Read the model definition and answer for the solid it produces. Units are mm, in the model's axes. Face numbers are marked on the shaded views. Coordinates: 2 decimals unless noted, no trailing zeros. Order: outer loops, then holes, each group sorted by start corner. A loop starts at its lowest first (then second) coordinate and runs counter-clockwise, first axis right, second up. Notation, with made-up numbers: M 87,-27.75 L 116,-27.75 A16 ccw 116,-12.75 Z; hole C -15,-17 d5. An arc over 180 degrees is marked long. Put each result on its own line as item: value.
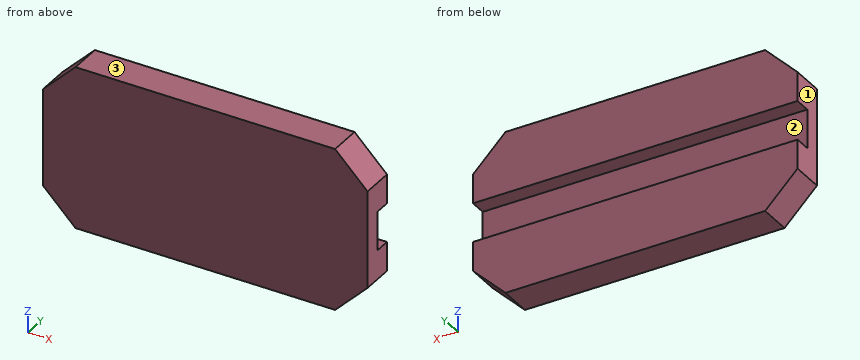
from build123d import *

# Parameters (mm, degrees)
SKETCH1_W           = 100
SKETCH1_H           = 50
BOSS_EXTRUDE1_DEPTH = 10
CHAMFER1_SIZE       = 10
SKETCH2_W           = 113.165724781
SKETCH2_H           = 12
CUT_EXTRUDE1_DEPTH  = 5


with BuildPart() as part:
    # Sketch1 → Boss-Extrude1 (new body)
    with BuildSketch(Plane(origin=(0, 0, 0), x_dir=(1, 0, 0), z_dir=(0, 1, 0))):
        Rectangle(SKETCH1_W, SKETCH1_H)
    extrude(amount=BOSS_EXTRUDE1_DEPTH)

    # Chamfer1
    chamfer1_edges = [part.edges().sort_by_distance(p)[0] for p in [
        (-50, 5, -25),
        (50, 5, -25),
        (50, 5, 25),
        (-50, 5, 25),
    ]]
    chamfer(chamfer1_edges, length=CHAMFER1_SIZE)

    # Sketch2 → Cut-Extrude1 (cut)
    with BuildSketch(Plane(origin=(0, 10, 0), x_dir=(1, 0, 0), z_dir=(0, 1, 0))):
        with Locations((-1.797960114, 0)):
            Rectangle(SKETCH2_W, SKETCH2_H)
    extrude(amount=-CUT_EXTRUDE1_DEPTH, mode=Mode.SUBTRACT)


solid = part.part
Q1. Find section D-D on y = 1. Write down the section's boundary in (x, z), plus the area to 3 significant figures.
Answers below:
outline: M -50,-15 L -40,-25 L 40,-25 L 50,-15 L 50,15 L 40,25 L -40,25 L -50,15 Z
area: 4,800 mm^2
Q2. Find section B-B on x = 41. Write down the section's boundary in (y, z).
Answers below:
outline: M 0,-24 L 10,-24 L 10,-6 L 5,-6 L 5,6 L 10,6 L 10,24 L 0,24 Z
Q3. Given pin 1 (3 mm diameter, centred on y = 8.5, z = 18.5, fed in from -X); pin 2 (3.5 mm diameter, centred on x = -21, z = 2, fed in from +Y); pin 3 (3 mm diameter, centred on y = 3.5, z = -18, fed in from +X), each flat-ended and moving along its own axis, determine where each tip first touches the part or whether it passes through.
Answers below:
pin 1: stops at x = -48
pin 2: stops at y = 5
pin 3: stops at x = 48.5
Q4. For a pull along Z with two mould halves and no side action, classify the marked faces 1, 2 and 3 as +Z half, -Z half, draft (parallel to the pull), parting line (faces both ways), or undercut.
Answers below:
face 1: draft
face 2: undercut
face 3: +Z half
Q5. Consider line 1 along Z through (x, y) = (33.5, 8.75); line 2 along Y through (x, z) = (-27, 3); line 3 along X through (y, z) = (3, 19). Determine where each line is inside the solid, lowest interval first.
Answers below:
line 1: z = -25 to -6, 6 to 25
line 2: y = 0 to 5
line 3: x = -46 to 46
Q6. Find section C-C on z = 17. Write down the section's boundary in (x, y), plus the area to 3 significant figures.
Answers below:
outline: M -48,0 L 48,0 L 48,10 L -48,10 Z
area: 960 mm^2
Q7. Find section A-A on y = 6. Write down the section's boundary in (x, z), plus the area to 3 significant figures.
Answers below:
outline: M -50,-15 L -40,-25 L 40,-25 L 50,-15 L 50,-6 L -50,-6 Z; M -50,6 L 50,6 L 50,15 L 40,25 L -40,25 L -50,15 Z
area: 3,600 mm^2
